from build123d import *

# Parameters (mm, degrees)
F0_R     = 9.525
F0_R_2   = 24.281079
F0_R_3   = 9.831352
F1_DEPTH = 12.7


with BuildPart() as f1:
    # F0 (on Front) → F1 (new body)
    with BuildSketch(Plane.XZ):
        with BuildLine():
            Line((-308.675736, 182.516785), (-308.675736, 55.516785))
            Line((-308.675736, 55.516785), (-194.375736, 55.516785))
            Line((-194.375736, 55.516785), (-158.488057, 19.238039))
            Line((-158.488057, 19.238039), (-22.676105, -118.053854))
            ThreePointArc((-22.676105, -118.053854), (-0.30253, -121.93622), (21.652907, -116.138945))
            Line((21.652907, -116.138945), (195.179168, 55.516785))
            Line((195.179168, 55.516785), (309.479168, 55.516785))
            Line((309.479168, 55.516785), (309.479168, 182.516785))
            Line((309.479168, 182.516785), (-308.675736, 182.516785))
        make_face()
        with Locations((-53.848, 30.116785)):
            Circle(F0_R, mode=Mode.SUBTRACT)
        with Locations((0, -58.783215)):
            Circle(F0_R, mode=Mode.SUBTRACT)
        with BuildLine():
            ThreePointArc((53.848, 20.591785), (47.112808, 36.851977), (63.373, 30.116785))
            ThreePointArc((63.373, 30.116785), (60.583192, 23.381593), (53.848, 20.591785))
        make_face(mode=Mode.SUBTRACT)
        with Locations((-64.168158, 119.016785)):
            Circle(F0_R_2, mode=Mode.SUBTRACT)
        with Locations((124.374732, 87.266785)):
            Circle(F0_R, mode=Mode.SUBTRACT)
        with Locations((124.374732, 150.766785)):
            Circle(F0_R, mode=Mode.SUBTRACT)
        with Locations((215.231842, 119.016785)):
            Circle(F0_R_3, mode=Mode.SUBTRACT)
    extrude(amount=F1_DEPTH)


solid = f1.part
Could you check a few things on this model? Use its own coordinates, in mm. A direction names the side the tool comes from. Coordinates: 2 decimals unless noted, no trailing zeros. Write each loop counter-clockwise with the first axis right and the second up, starting at its lowest first coordinate (ties: lowest second). Pieces come first, ordered by that corner, then holes. Notation, with made-up numbers: (-36, -23.5) - (-6, -23.5) arc R23 ccw to (-6, -10.5) - close; hole circle Ø3 at (28, -37.5). An arc over 180 degrees is marked (long way). Put each result on its own line as item: value. Start each with the question number.
Q1. I want a section at A-A on x = 0. Write out the boundary of the cut face in (y, z), plus the area to 3 significant figures.
Q2. I want a section at C-C on z = 10. Write out the boundary of the cut face in (x, y), plus the area to 3 significant figures.
Q3. I want a section at D-D on x = -214. Write out the boundary of the cut face in (y, z).
Q4. Please list where these lines run through material, in increasing order: L1, parallel to X at y = -10.75, z = 119; L2, parallel to X at y = -11.25, z = 37.5; L3, parallel to Z at x = 215, y = -7.
Q5. I'm going to push flat-ended pins straight in: P1, Ø12, axis at x = 215.23, z = 119.02, coming from the -Y side; P2, Ø6.5, axis at x = 264, y = -8.5, coming from the -Z side; P3, Ø1, axis at x = -170.5, y = -2.5, coming from the -Z side; P4, Ø3, axis at x = 126.5, y = -2.5, coming from the -Z side. Where does each tip first touch, or does it pass through?
Q6. I want a section at B-B on y = -5.5. Write out the boundary of the cut face in (x, z) (3 decimals), plus the area to 3 significant figures.
Q7. Which directions (+Z, -Z, +X, -X, +Y, -Y) give clear straight access to the entire face, cutting with the end or side of a thin tool? Please do faces 1 (the flat face through (-308.676, -6, 120)), 2 (the flat face through (-252, -6, 55.517)).
Q8. Thinking about a two-plate mould opening in Z: for faces 3 (the flat face through (5, -6, 182.517)), 4 (the cylindrical face through (116.816, -6.261, 81.471)), 5 (the flat face through (-4, -12.7, 66)), 6 (the flat face through (252, -6, 55.517)), which applies, pulls with the +Z half, pulls with the -Z half, needs draft (parallel to the pull), parting line crosses it, or undercut?
Checks:
1. outline: (-12.7, -121.92) - (0, -121.92) - (0, -68.31) - (-12.7, -68.31) - close; (-12.7, -49.26) - (0, -49.26) - (0, 182.52) - (-12.7, 182.52) - close
1. area: 3,620 mm²
2. outline: (-149.35, -12.7) - (149.17, -12.7) - (149.17, 0) - (-149.35, 0) - close
2. area: 3,790 mm²
3. outline: (-12.7, 55.52) - (0, 55.52) - (0, 182.52) - (-12.7, 182.52) - close
4. L1: -308.68 to -88.45, -39.89 to 205.4, 225.06 to 309.48
4. L2: -176.55 to -59.87, -47.83 to 47.83, 59.87 to 176.97
4. L3: 55.52 to 109.19, 128.85 to 182.52
5. P1: through
5. P2: z = 55.52
5. P3: z = 30.88
5. P4: z = -13.91
6. outline: (-308.676, 55.517) - (-194.376, 55.517) - (-22.676, -118.054) arc R53.222 ccw to (21.653, -116.139) - (195.179, 55.517) - (309.479, 55.517) - (309.479, 182.517) - (-308.676, 182.517) - close; hole circle Ø48.562 at (-64.168, 119.017); hole circle Ø19.05 at (-53.848, 30.117); hole circle Ø19.05 at (0, -58.783); hole circle Ø19.05 at (53.848, 30.117); hole circle Ø19.05 at (124.375, 87.267); hole circle Ø19.05 at (124.375, 150.767); hole circle Ø19.663 at (215.232, 119.017)
6. area: 113,000 mm²
7. face 1: +Z, -Z, -X, +Y, -Y
7. face 2: -Z, -X, +Y, -Y
8. face 3: pulls with the +Z half
8. face 4: undercut
8. face 5: needs draft
8. face 6: pulls with the -Z half
